Geometry check sheet. Reference: the model listing, model coordinates, mm. Face numbers are marked on the shaded views. A direction names the side the tool comes from. Coordinates: 2 decimals unless noted, no trailing zeros. Loops run counter-clockwise (first coordinate to the right, second up) from the corner with the lowest first, then second, coordinate; pieces in that order, holes last.
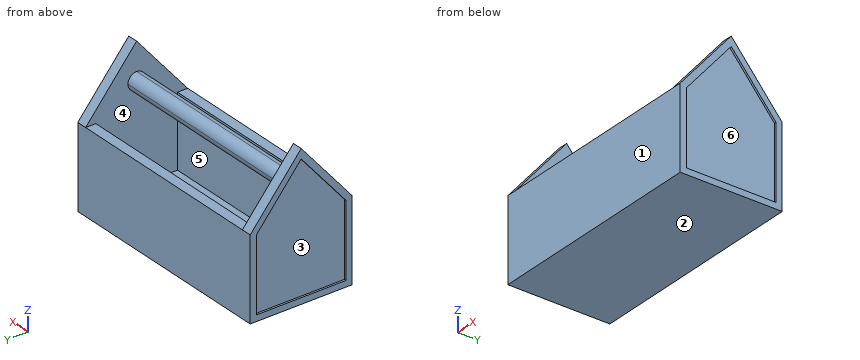
from build123d import *

# Parameters (mm, degrees)
F0_W      = 110
F0_H      = 50
F1_DEPTH  = 5
F2_W      = 5
F2_H      = 40
F3_DEPTH  = 35
F5_DEPTH  = 5
F7_DEPTH  = 5
F9_DEPTH  = 101
F11_DEPTH = 1
F13_DEPTH = 1


with BuildPart() as f1:
    # F0 (on Top) → F1 (new body)
    with BuildSketch(Plane.XY):
        with Locations((4.572784, -5.880122)):
            Rectangle(F0_W, F0_H)
    extrude(amount=F1_DEPTH)

    # F2 (on face) → F3 (join)
    with BuildSketch(Plane.XY.offset(5)):
        Polygon((59.572784, 19.119878), (-50.427216, 19.119878), (-50.427216, 14.119878), (-45.427216, 14.119878), (54.572784, 14.119878), (59.572784, 14.119878), align=None)
        with Locations((-47.927216, -5.880122)):
            Rectangle(F2_W, F2_H)
        with Locations((57.072784, -5.880122)):
            Rectangle(F2_W, F2_H)
        Polygon((-45.427216, -25.880122), (-50.427216, -25.880122), (-50.427216, -30.880122), (59.572784, -30.880122), (59.572784, -25.880122), (54.572784, -25.880122), align=None)
    extrude(amount=F3_DEPTH)

    # F4 (on face) → F5 (join)
    with BuildSketch(Plane(origin=(-50.427216, 0, 0), x_dir=(0, -1, 0), z_dir=(-1, 0, 0))):
        Polygon((30.880122, 40), (5.880122, 70), (5.880122, 40), align=None)
        Polygon((5.880122, 70), (-19.119878, 40), (5.880122, 40), align=None)
    extrude(amount=-F5_DEPTH)

    # F6 (on face) → F7 (join)
    with BuildSketch(Plane.YZ.offset(59.572784)):
        Polygon((-30.880122, 40), (-5.880122, 40), (-5.880122, 70), align=None)
        Polygon((-5.880122, 70), (-5.880122, 40), (19.119878, 40), align=None)
    extrude(amount=-F7_DEPTH)

    # F8 (on face) → F9 (join)
    with BuildSketch(Plane.YZ.offset(-45.427216)):
        with BuildLine():
            ThreePointArc((-1.630122, 52.12112), (-2.874919, 55.126323), (-5.880122, 56.37112))
            Line((-5.880122, 56.37112), (-5.880122, 47.87112))
            ThreePointArc((-5.880122, 47.87112), (-2.874919, 49.115916), (-1.630122, 52.12112))
        make_face()
        with BuildLine():
            Line((-5.880122, 47.87112), (-5.880122, 56.37112))
            ThreePointArc((-5.880122, 56.37112), (-10.130122, 52.12112), (-5.880122, 47.87112))
        make_face()
    extrude(amount=F9_DEPTH)

    # F10 (on face) → F11 (cut)
    with BuildSketch(Plane.YZ.offset(59.572784)):
        Polygon((-27.880122, 38.91385), (-27.880122, 3), (16.119878, 3), (16.119878, 38.91385), (-5.880122, 65.31385), align=None)
    extrude(amount=-F11_DEPTH, mode=Mode.SUBTRACT)

    # F12 (on face) → F13 (cut)
    with BuildSketch(Plane(origin=(-50.427216, 0, 0), x_dir=(0, -1, 0), z_dir=(-1, 0, 0))):
        Polygon((-16.119878, 38.91385), (-16.119878, 3), (27.880122, 3), (27.880122, 38.91385), (5.880122, 65.31385), align=None)
    extrude(amount=-F13_DEPTH, mode=Mode.SUBTRACT)


solid = f1.part
1) Access from +Z, -Z, +X, -X, +Y, -Y to the whole of each face (thin tool, end or side, straight path). Record for the marked faces 4, 5 and 6.
Data:
face 4: none
face 5: +Z
face 6: +X
2) Section check A-A on x = -23.5. Record the cut outline in (y, z).
Data:
outline: (-30.88, 0) - (19.12, 0) - (19.12, 40) - (14.12, 40) - (14.12, 5) - (-25.88, 5) - (-25.88, 40) - (-30.88, 40) - close; (-5.88, 47.87) arc R4.25 ccw to (-1.63, 52.12) arc R4.25 ccw to (-5.88, 56.37) arc R4.25 ccw to start
3) Section check B-B on z = 29. Record the cut outline in (x, y), and give its area (3 significant figures).
Data:
outline: (-50.43, -30.88) - (59.57, -30.88) - (59.57, -27.88) - (58.57, -27.88) - (58.57, 16.12) - (59.57, 16.12) - (59.57, 19.12) - (-50.43, 19.12) - (-50.43, 16.12) - (-49.43, 16.12) - (-49.43, -27.88) - (-50.43, -27.88) - close; hole (-45.43, -25.88) - (54.57, -25.88) - (54.57, 14.12) - (-45.43, 14.12) - close
area: 1,410 mm2
4) Mould release check, pull along Y, two halves, no side actions. Record for the marked faces 1, 2 and 3: +Y half, -Y half, draft (parallel to the pull), parting line (faces both ways), or undercut.
Data:
face 1: -Y half
face 2: draft
face 3: undercut
5) Section check D-D on y = -22. Record the cut outline in (x, z), and give its area (3 significant figures).
Data:
outline: (-50.43, 0) - (59.57, 0) - (59.57, 3) - (58.57, 3) - (58.57, 45.97) - (59.57, 45.97) - (59.57, 50.66) - (54.57, 50.66) - (54.57, 5) - (-45.43, 5) - (-45.43, 50.66) - (-50.43, 50.66) - (-50.43, 45.97) - (-49.43, 45.97) - (-49.43, 3) - (-50.43, 3) - close
area: 921 mm2
6) Material ranges on probe 1 along X at (y, z) = (-6, 11); probe 2 along Y at (x, z) = (-31, 5.5); probe 3 along Z at (x, y) = (36, 8.5), recorded low to high.
Data:
probe 1: x = -49.43 to -45.43, 54.57 to 58.57
probe 2: y = -30.88 to -25.88, 14.12 to 19.12
probe 3: z = 0 to 5
7) Depth check by flat-ended pin: pin 1 (8 mm diameter, centred on x = 7, y = -9.5, fed in from +Z); pin 2 (25 mm diameter, centred on y = -8, z = 37.5, fed in from -X); pin 3 (4 mm diameter, centred on x = 22.5, y = 17, fed in from +Z). Enter the tip coordinate at first touch or a pass-through.
Data:
pin 1: stops at z = 56.37
pin 2: stops at x = -49.43
pin 3: stops at z = 40
8) Section check C-C on y = -3. Record the cut outline in (x, z).
Data:
outline: (-50.43, 0) - (59.57, 0) - (59.57, 3) - (58.57, 3) - (58.57, 61.86) - (59.57, 61.86) - (59.57, 66.54) - (54.57, 66.54) - (54.57, 55.25) - (-45.43, 55.25) - (-45.43, 66.54) - (-50.43, 66.54) - (-50.43, 61.86) - (-49.43, 61.86) - (-49.43, 3) - (-50.43, 3) - close; hole (-45.43, 5) - (54.57, 5) - (54.57, 49) - (-45.43, 49) - close
